For this review, take the finished solid that the model builds, in its own axes (mm). A direction names the side the tool comes from. Round coordinates to 2 decimals unless told otherwise and drop trailing zeros. Loops run counter-clockwise (first coordinate to the right, second up) from the corner with the lowest first, then second, coordinate; pieces in that order, holes last.
1) Tool access review of faces 1 (the cylindrical face through (53.198, 176.478, 78.404)), 2 (the flat face through (3, 180.534, -66)), 3 (the flat face through (3, 190, -62)), 4 (the flat face through (-27, 157, 40)): name each direction out of +Z, -Z, +X, -X, +Y, -Y from which nothing blocks a thin tool from reaching the whole face with its end or side.
2) Take a section at B-B (x = 5). Give the number of separate pieces and of enclosed holes in the cut face, then the cut area to 3 significant figures.
3) Take a section at C-C (z = -33.5). State the section outline as (x, y) points, then the cut area to 3 significant figures.
4) Wall thickness on L1, parallel to Z at x = -185.5, y = 131; L2, parallel to Z at x = 75, y = 154.5; L3, parallel to Y at x = 85.5, z = -58: over which ranges is each line inside the solid? List them lowest first.
5) Insertion check: pin 1 (5.5 mm diameter, centred on y = 166.5, z = -59, fed in from +X); pin 2 (19 mm diameter, centred on x = -145, z = 72.68, fed in from +Y); pin 3 (1.6 mm diameter, centred on x = 51.5, y = 189, fed in from -Z). Each pin has a flat end and moves straight along its axis. Give the tip position at first contact, or say it passes through.
6) Mouldability with a two-part tool opening along X and no side actions: class faces 5 (the flat face through (212.5, 179, -1)), 6 (the flat face through (-27, 142, -6)), 7 (the cylindrical face through (3.198, 176.478, 78.404)) as pulls with the +X half, pulls with the -X half, needs draft (parallel to the pull), parting line crosses it, or undercut.
7) Take a section at A-A (x = 186). State the section outline as (y, z) points.
```python
from build123d import *

# Parameters (mm, degrees)
BOSS_EXTRUDE1_DEPTH             = 212.5
BOSS_EXTRUDE1_DEPTH_BACK        = 212.5
SKETCH3_R                       = 6
CUT_EXTRUDE1_DEPTH              = 299.531180557
FILLET1_R                       = 1
BOSS_EXTRUDE2_DEPTH             = 150
BOSS_EXTRUDE2_DEPTH_BACK        = 200
SKETCH4_W                       = 5
SKETCH4_H                       = 12
SKETCH4_H_2                     = 30
SKETCH4_H_3                     = 45
SKETCH4_H_4                     = 60
BOSS_EXTRUDE3_REACH             = 300.248
SKETCH5_W                       = 5
SKETCH5_H                       = 15
BOSS_EXTRUDE3_DIRECTION_2_REACH = 300.248
BOSS_EXTRUDE4_DEPTH             = 180
BOSS_EXTRUDE4_DEPTH_BACK        = 180
SKETCH6_W                       = 5
SKETCH6_H                       = 10
CUT_EXTRUDE2_DEPTH              = 175
CUT_EXTRUDE2_DEPTH_BACK         = 165
SKETCH7_W                       = 20
SKETCH7_H                       = 7


with BuildPart() as part:
    # Sketch2 → Boss-Extrude1 (new, two sides: drawn at the far end of the back side and taken through both)
    with BuildSketch(Plane(origin=(0, 0, 0), x_dir=(0, 0, -1), z_dir=(1, 0, 0)).offset(-BOSS_EXTRUDE1_DEPTH_BACK)):
        with BuildLine():
            Line((-87.681240867, 172.53405461), (-93.974488101, 180.03405461))
            ThreePointArc((-93.974488101, 180.03405461), (0, 187.439087042), (93.974488101, 180.03405461))
            Line((93.974488101, 180.03405461), (87.681240867, 172.53405461))
            Line((87.681240867, 172.53405461), (-87.681240867, 172.53405461))
        make_face()
    extrude(amount=BOSS_EXTRUDE1_DEPTH + BOSS_EXTRUDE1_DEPTH_BACK)

    # Sketch3 → Cut-Extrude1 (cut, through all)
    with BuildSketch(Plane(origin=(0, 0, 0), x_dir=(1, 0, 0), z_dir=(0, 1, 0))):
        with Locations(Location((-145, 72.681240867, 0), (0, 0, 90))):
            Circle(SKETCH3_R)
        with Locations(Location((-95, 72.681240867, 0), (0, 0, 90))):
            Circle(SKETCH3_R)
        with Locations(Location((-45, 72.681240867, 0), (0, 0, 90))):
            Circle(SKETCH3_R)
        with Locations(Location((5, 72.681240867, 0), (0, 0, 90))):
            Circle(SKETCH3_R)
        with Locations(Location((55, 72.681240867, 0), (0, 0, 90))):
            Circle(SKETCH3_R)
        with Locations(Location((105, 72.681240867, 0), (0, 0, 90))):
            Circle(SKETCH3_R)
        with Locations(Location((155, 72.681240867, 0), (0, 0, 90))):
            Circle(SKETCH3_R)
    cut_extrude1 = extrude(amount=CUT_EXTRUDE1_DEPTH, mode=Mode.SUBTRACT)

    # Mirror1: Cut-Extrude1 across plane
    add(cut_extrude1.mirror(Plane.XY), mode=Mode.SUBTRACT)

    # Fillet1
    fillet1_edges = [part.edges().sort_by_distance(p)[0] for p in [
        (0, 180.03405461, 93.974488101),
        (0, 180.03405461, -93.974488101),
    ]]
    fillet(fillet1_edges, radius=FILLET1_R)

    # Sketch4 → Boss-Extrude2 (add, two sides: drawn at the far end of the back side and taken through both)
    with BuildSketch(Plane(origin=(0, 0, 0), x_dir=(0, 0, -1), z_dir=(1, 0, 0)).offset(-BOSS_EXTRUDE2_DEPTH_BACK)):
        with Locations((-59.5, 166.53405461)):
            Rectangle(SKETCH4_W, SKETCH4_H)
        with Locations((-42.5, 157.53405461)):
            Rectangle(SKETCH4_W, SKETCH4_H_2)
        with Locations((-25.5, 150.03405461)):
            Rectangle(SKETCH4_W, SKETCH4_H_3)
        with Locations((-8.5, 142.53405461)):
            Rectangle(SKETCH4_W, SKETCH4_H_4)
        with Locations((8.5, 142.53405461)):
            Rectangle(SKETCH4_W, SKETCH4_H_4)
        with Locations((25.5, 150.03405461)):
            Rectangle(SKETCH4_W, SKETCH4_H_3)
        with Locations((59.5, 166.53405461)):
            Rectangle(SKETCH4_W, SKETCH4_H)
        with Locations((42.5, 157.53405461)):
            Rectangle(SKETCH4_W, SKETCH4_H_2)
    extrude(amount=BOSS_EXTRUDE2_DEPTH + BOSS_EXTRUDE2_DEPTH_BACK)

    # Boss-Extrude3: up to this face of the body (flat: up to its plane)
    boss_extrude3_end = Plane(part.part.faces().sort_by_distance((212.5, 179.031198014, 0))[0])
    # Sketch5 → Boss-Extrude3 (add, up to the picked face)
    with BuildSketch(Plane(origin=(0, 0, 0), x_dir=(0, 0, -1), z_dir=(1, 0, 0)), mode=Mode.PRIVATE) as boss_extrude3_sk1:
        with Locations((-59.5, 187.53405461)):
            Rectangle(SKETCH5_W, SKETCH5_H)
    boss_extrude3_tool1 = split(extrude(boss_extrude3_sk1.sketch, amount=BOSS_EXTRUDE3_REACH, mode=Mode.PRIVATE), bisect_by=boss_extrude3_end, keep=Keep.BOTH, mode=Mode.PRIVATE)
    # Sketch5 → Boss-Extrude3 (add, up to the picked face)
    with BuildSketch(Plane(origin=(0, 0, 0), x_dir=(0, 0, -1), z_dir=(1, 0, 0)), mode=Mode.PRIVATE) as boss_extrude3_sk2:
        with Locations((59.5, 187.53405461)):
            Rectangle(SKETCH5_W, SKETCH5_H)
    boss_extrude3_tool2 = split(extrude(boss_extrude3_sk2.sketch, amount=BOSS_EXTRUDE3_REACH, mode=Mode.PRIVATE), bisect_by=boss_extrude3_end, keep=Keep.BOTH, mode=Mode.PRIVATE)
    add(boss_extrude3_tool1.solids().sort_by(Axis((0, 187.534055, 59.5), (1, 0, 0)))[0])
    add(boss_extrude3_tool2.solids().sort_by(Axis((0, 187.534055, -59.5), (1, 0, 0)))[0])

    # Boss-Extrude3 direction 2: up to this face of the body (flat: up to its plane)
    boss_extrude3_direction_2_end = Plane(part.part.faces().sort_by_distance((-212.5, 179.031198014, 0))[0])
    # Sketch5 → Boss-Extrude3 direction 2 (add, up to the picked face)
    with BuildSketch(Plane(origin=(0, 0, 0), x_dir=(0, 0, -1), z_dir=(1, 0, 0)), mode=Mode.PRIVATE) as boss_extrude3_direction_2_sk1:
        with Locations((-59.5, 187.53405461)):
            Rectangle(SKETCH5_W, SKETCH5_H)
    boss_extrude3_direction_2_tool1 = split(extrude(boss_extrude3_direction_2_sk1.sketch, amount=-BOSS_EXTRUDE3_DIRECTION_2_REACH, mode=Mode.PRIVATE), bisect_by=boss_extrude3_direction_2_end, keep=Keep.BOTH, mode=Mode.PRIVATE)
    # Sketch5 → Boss-Extrude3 direction 2 (add, up to the picked face)
    with BuildSketch(Plane(origin=(0, 0, 0), x_dir=(0, 0, -1), z_dir=(1, 0, 0)), mode=Mode.PRIVATE) as boss_extrude3_direction_2_sk2:
        with Locations((59.5, 187.53405461)):
            Rectangle(SKETCH5_W, SKETCH5_H)
    boss_extrude3_direction_2_tool2 = split(extrude(boss_extrude3_direction_2_sk2.sketch, amount=-BOSS_EXTRUDE3_DIRECTION_2_REACH, mode=Mode.PRIVATE), bisect_by=boss_extrude3_direction_2_end, keep=Keep.BOTH, mode=Mode.PRIVATE)
    add(boss_extrude3_direction_2_tool1.solids().sort_by(Axis((0, 187.534055, 59.5), (-1, 0, 0)))[0])
    add(boss_extrude3_direction_2_tool2.solids().sort_by(Axis((0, 187.534055, -59.5), (-1, 0, 0)))[0])

    # Sketch6 → Boss-Extrude4 (add, two sides: drawn at the far end of the back side and taken through both)
    with BuildSketch(Plane(origin=(0, 0, 0), x_dir=(0, 0, -1), z_dir=(1, 0, 0)).offset(-BOSS_EXTRUDE4_DEPTH_BACK)):
        with Locations((-42.5, 185.03405461)):
            Rectangle(SKETCH6_W, SKETCH6_H)
        with Locations((-25.5, 185.03405461)):
            Rectangle(SKETCH6_W, SKETCH6_H)
        with Locations((-8.5, 185.03405461)):
            Rectangle(SKETCH6_W, SKETCH6_H)
        with Locations((8.5, 185.03405461)):
            Rectangle(SKETCH6_W, SKETCH6_H)
        with Locations((25.5, 185.03405461)):
            Rectangle(SKETCH6_W, SKETCH6_H)
        with Locations((42.5, 185.03405461)):
            Rectangle(SKETCH6_W, SKETCH6_H)
    extrude(amount=BOSS_EXTRUDE4_DEPTH + BOSS_EXTRUDE4_DEPTH_BACK)

    # Sketch7 → Cut-Extrude2 (cut, two sides: drawn at the far end of the back side and taken through both)
    with BuildSketch(Plane(origin=(0, 0, 0), x_dir=(0, 0, -1), z_dir=(1, 0, 0)).offset(-CUT_EXTRUDE2_DEPTH_BACK)):
        with Locations((-72.318759133, 184.03405461)):
            Rectangle(SKETCH7_W, SKETCH7_H)
        with Locations((72.681240867, 184.03405461)):
            Rectangle(SKETCH7_W, SKETCH7_H)
    extrude(amount=CUT_EXTRUDE2_DEPTH + CUT_EXTRUDE2_DEPTH_BACK, mode=Mode.SUBTRACT)


solid = part.part
```
Response:
1. face 1: +Y, -Y
1. face 2: +Y
1. face 3: -Z, +X, -X, +Y
1. face 4: +X, -X, -Y
2. separate pieces: 3
2. enclosed holes: 0
2. area: 3,670 mm2
3. outline: (-212.5, 172.53) - (212.5, 172.53) - (212.5, 186.5) - (-212.5, 186.5) - close
3. area: 5,940 mm2
4. L1: z = -28 to -23, -11 to -6, 6 to 11, 23 to 28
4. L2: z = -45 to -40, -28 to -23, -11 to -6, 6 to 11, 23 to 28, 40 to 45
4. L3: y = 160.53 to 195.03
5. pin 1: stops at x = 150
5. pin 2: stops at y = 180.53
5. pin 3: stops at z = -62
6. face 5: pulls with the +X half
6. face 6: needs draft
6. face 7: undercut
7. outline: (172.53, -87.68) - (178.68, -92.84) arc R1 ccw to (180.31, -92.22) arc R600 ccw to (184.23, -62) - (195.03, -62) - (195.03, -57) - (184.73, -57) arc R600 ccw to (184.73, 57) - (195.03, 57) - (195.03, 62) - (184.23, 62) arc R600 ccw to (180.31, 92.22) arc R1 ccw to (178.68, 92.84) - (172.53, 87.68) - close
